Work out the finished part from the listing and answer in its coordinate system (mm). Face numbers are marked on the shaded views. A direction names the side the tool comes from. Round coordinates to 2 decimals unless told otherwise and drop trailing zeros. Order: outer loops, then holes, each group sorted by start corner. A loop starts at its lowest first (then second) coordinate and runs counter-clockwise, first axis right, second up. Notation, with made-up numbers: M 13,64 L 47,64 A8 ccw 47,79 Z; hole C 20.5,-21.75 d2. An arc over 180 degrees is marked long. Return JSON: item names as keys, results as strings.
from build123d import *

# Parameters (mm, degrees)
F0_R            = 28.575
F1_DEPTH        = 50.8
F2_R            = 25.4
F3_DEPTH        = 25.4
F5_DEPTH        = 6.35
F5_DEPTH_BACK   = 6.35
F5_COPIES_COUNT = 6
F6_R            = 6.35
F7_DEPTH        = 25.4
F7_COPIES_COUNT = 6


# Not quite as in the source:
# - a pattern or mirror of a feature is missing from the dataset's text; its kind, count and spacing are read off the source's solid


with BuildPart() as f1:
    # F0 (on Top) → F1 (new body)
    with BuildSketch(Plane.XY):
        Circle(F0_R)
    extrude(amount=F1_DEPTH)

    # F2 (on face) → F3 (cut)
    with BuildSketch(Plane(origin=(0, 0, 0), x_dir=(1, 0, 0), z_dir=(0, 0, -1))):
        Circle(F2_R)
    extrude(amount=-F3_DEPTH, mode=Mode.SUBTRACT)

    # F4 (on Front) → F5 (join, two sides)
    with BuildSketch(Plane.XZ) as f5_sk:
        with BuildLine():
            ThreePointArc((-28.718591857, 50.8), (-54.118591857, 25.4), (-28.718591857, 0))
            Line((-28.718591857, 0), (-22.9244896994, 0))
            Line((-22.9244896994, 0), (-22.9244896994, 50.8))
            Line((-22.9244896994, 50.8), (-28.718591857, 50.8))
        make_face()
    f5 = extrude(amount=F5_DEPTH) + extrude(f5_sk.sketch, amount=-F5_DEPTH_BACK)

    # F5_copies: F5 ×6 about axis
    f5_copies_axis = Axis((0, 0, 0), (0, 0, 1))
    for i in range(1, F5_COPIES_COUNT):
        add(f5.rotate(f5_copies_axis, i * 360 / F5_COPIES_COUNT))

    # F6 (on face) → F7 (cut)
    with BuildSketch(Plane.XZ.offset(6.35)):
        with Locations((-38.02051193, 25.4)):
            Circle(F6_R)
    f7 = extrude(amount=-F7_DEPTH, mode=Mode.SUBTRACT)

    # F7_copies: F7 ×6 about axis
    f7_copies_axis = Axis((0, 0, 0), (0, 0, 1))
    for i in range(1, F7_COPIES_COUNT):
        add(f7.rotate(f7_copies_axis, i * 360 / F7_COPIES_COUNT), mode=Mode.SUBTRACT)


solid = f1.part
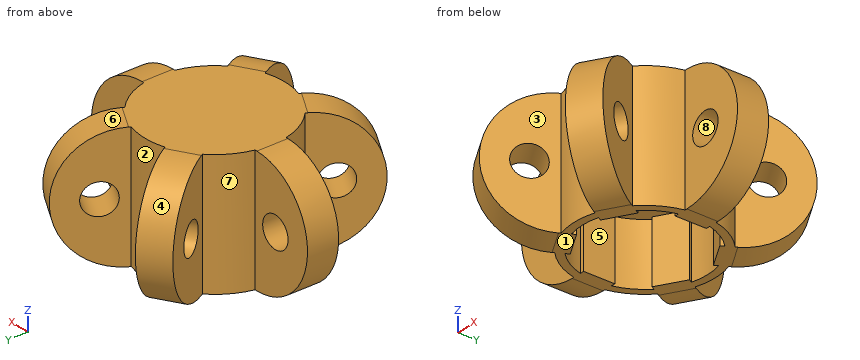
Item 1: Find section A-A (y = -4.5). Determine the outline of the cut face in (x, z).
Output:
{"outline": "M -28.72,0 L -22.92,0 L -22.92,25.4 L 22.92,25.4 L 22.92,0 L 28.72,0 A25.4 ccw 28.72,50.8 L -28.72,50.8 A25.4 ccw Z; hole C -38.02,25.4 d12.7; hole C 38.02,25.4 d12.7"}
Item 2: Each of these flat-tipped pins is pushed along its axis until it touches: pin 1 (21 mm diameter, centred on x = -41, z = 34.5, fed in from -Y); pin 2 (8 mm diameter, centred on y = -33, z = 26.5, fed in from -X); pin 3 (16.5 mm diameter, centred on x = 38.02, z = 25.4, fed in from -Y). Where does it stop, or does it pass through?
Output:
{"pin 1": "stops at y = -43.83", "pin 2": "stops at x = -28.69", "pin 3": "stops at y = -45.3"}
Item 3: Which of the six approach directions +Z, -Z, +X, -X, +Y, -Y give full straight-line access (tool end or side, diameter ignored) to the marked faces 5, 6, 7 and 8?
Output:
{"face 5": "-Z", "face 6": "+X, +Y", "face 7": "+Z, -Z, -X", "face 8": "none"}
Item 4: Find section D-D (y = 8). Determine the outline of the cut face in (x, z), plus the area to 3 significant figures.
Output:
{"outline": "M -27.43,0 L -24.11,0 L -24.11,25.4 L 24.11,25.4 L 24.11,0 L 27.43,0 L 27.43,50.8 L -27.43,50.8 Z", "area": "1,560 mm^2"}
Item 5: Find section B-B (x = -38.5). Determine the outline of the cut face in (y, z).
Output:
{"outline": "M -6.35,1.96 L 6.35,1.96 L 6.35,19.07 L -6.35,19.07 Z; M -6.35,31.73 L 6.35,31.73 L 6.35,48.84 L -6.35,48.84 Z"}
Item 6: Find section C-C (z = 38.5). Determine the outline of the cut face in (x, y) (3 decimals), plus the area to 3 significant figures.
Output:
{"outline": "M -50.48,-6.35 L -27.861,-6.35 A28.575 ccw -19.43,-20.953 L -30.739,-40.542 L -19.741,-46.892 L -8.431,-27.303 A28.575 ccw 8.431,-27.303 L 19.741,-46.892 L 30.739,-40.542 L 19.43,-20.953 A28.575 ccw 27.861,-6.35 L 50.48,-6.35 L 50.48,6.35 L 27.861,6.35 A28.575 ccw 19.43,20.953 L 30.739,40.542 L 19.741,46.892 L 8.431,27.303 A28.575 ccw -8.431,27.303 L -19.741,46.892 L -30.739,40.542 L -19.43,20.953 A28.575 ccw -27.861,6.35 L -50.48,6.35 Z", "area": "4,250 mm^2"}
Item 7: Consider line 1 along X through (y, z) = (-2, 25); line 2 along X through (y, z) = (18, 2); line 3 along Y through (x, z) = (21, 44). Determine where each line is inside the solid, lowest interval first. Write a range as [from, to].
Output:
{"line 1": "x = [-54.12, -44.36], [-31.68, -22.92], [22.92, 31.68], [44.36, 54.12]", "line 2": "x = [-22.19, -17.92], [-17.72, -14.67], [14.67, 17.72], [17.92, 22.19]", "line 3": "y = [-41.01, -23.67], [-19.38, 19.38], [23.67, 41.01]"}
Item 8: The mould has two halves that part along X. Classify the marked faces 1, 2, 3 and 4: pulls with the +X half, pulls with the -X half, needs draft (parallel to the pull), parting line crosses it, or undercut.
Output:
{"face 1": "needs draft", "face 2": "undercut", "face 3": "undercut", "face 4": "pulls with the -X half"}
